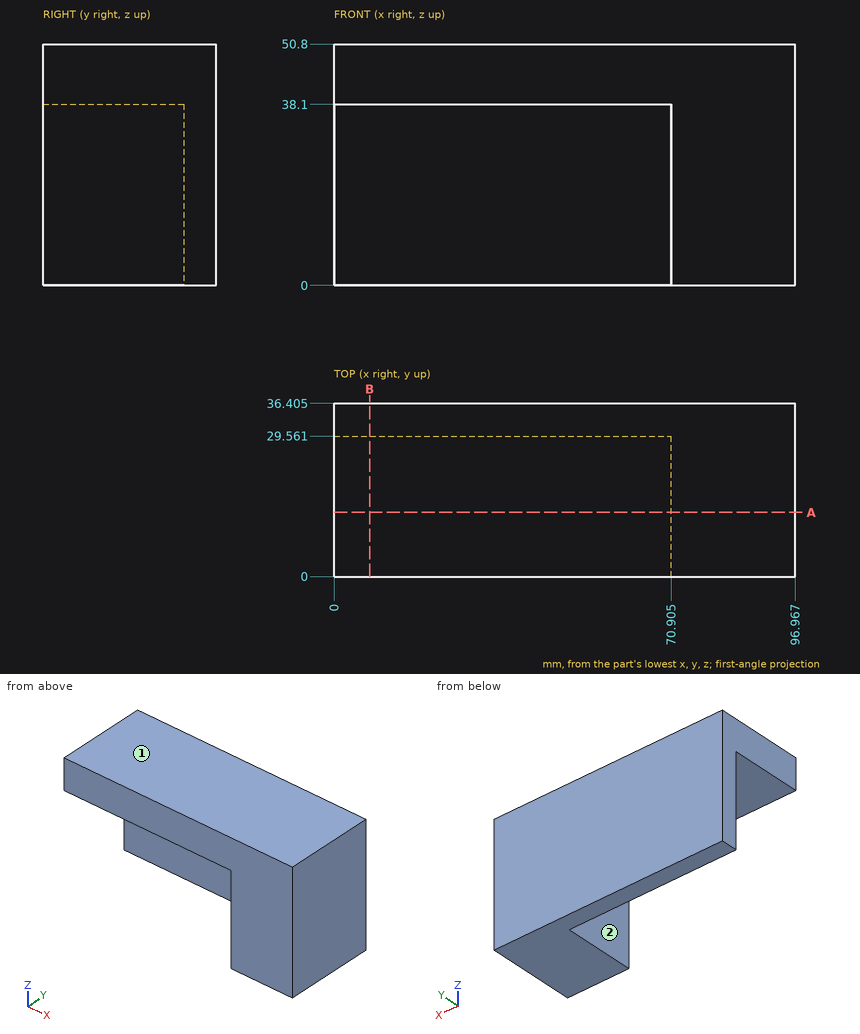
Source: three-view drawing plus pictorial views. Frame: mm from the lowest corner of the part. A direction names the side the tool comes from. Coordinates: 2 decimals unless noted, no trailing zeros. Write each loop counter-clockwise with the first axis right and the second up, starting at its lowest first coordinate (ties: lowest second). Pieces come first, ordered by that corner, then holes. Notation, with made-up numbers: (4, 55) - (55, 55) arc R12 cw to (55, 75) - close; hole circle Ø3 at (-10, -13.5). An arc over 180 degrees is marked (long way). Answer as a JSON object with one key per item and string values.
Q1. Material intervals for line 1 (X direction, y = 3.5, z = 2.5) (1 decimal); line 2 (Y direction, x = 20, z = 32) (1 decimal); line 3 (Z direction, x = 33.5, y = 20), sorted ascending. Write a range as [from, to].
Ans:
{"line 1": "x = [70.9, 97]", "line 2": "y = [29.6, 36.4]", "line 3": "z = [38.1, 50.8]"}
Q2. First-contact query: pin 1 Ø2 at (y, z) = (6.5, 22.5) entering from -X (1 decimal); pin 2 Ø11.5 at (x, z) = (38.5, 19.5) entering from -Y. Flat tips, straight axial feed; report the tip coordinate or a pass-through.
Ans:
{"pin 1": "stops at x = 70.9", "pin 2": "stops at y = 29.56"}
Q3. Section query A-A, the plane y = 13.5. Output: boundary loops of the cut face in (x, z) (1 decimal).
Ans:
{"outline": "(0, 38.1) - (70.9, 38.1) - (70.9, 0) - (97, 0) - (97, 50.8) - (0, 50.8) - close"}
Q4. Set-up query: the marked faces 1 and 2. Return all of +Z, -Z, +X, -X, +Y, -Y with unobstructed straight access to the full face (end or side cutting, diameter ignored); none if empty.
Ans:
{"face 1": "+Z, +X, -X, +Y, -Y", "face 2": "-Z, -X, -Y"}
Q5. Section query B-B, the plane x = 7.5. Output: boundary loops of the cut face in (y, z) (1 decimal).
Ans:
{"outline": "(0, 38.1) - (29.6, 38.1) - (29.6, 0) - (36.4, 0) - (36.4, 50.8) - (0, 50.8) - close"}
